from build123d import *

# Parameters (mm, degrees)
F1_DEPTH = 26
F2_R     = 3
F3_DEPTH = 25
F4_R     = 3
F5_DEPTH = 25
F6_R     = 4
F7_R     = 0.5


with BuildPart() as f1:
    # F0 (on Front) → F1 (new body)
    with BuildSketch(Plane.XZ):
        Polygon((0, 0), (0, 33.5), (-6.5, 33.5), (-6.5, -6.5), (19.5, -6.5), (19.5, 0), align=None)
    extrude(amount=-F1_DEPTH)

    # F2 (on Right) → F3 (cut)
    with BuildSketch(Plane.YZ):
        with Locations((13, 23.5)):
            Circle(F2_R)
    extrude(amount=-F3_DEPTH, mode=Mode.SUBTRACT)

    # F4 (on Top) → F5 (cut)
    with BuildSketch(Plane.XY):
        with Locations((6.5, 13)):
            Circle(F4_R)
    extrude(amount=-F5_DEPTH, mode=Mode.SUBTRACT)

    # F6
    f6_edges = [f1.edges().sort_by_distance(p)[0] for p in [
        (-6.5, 13, 33.5),
        (19.5, 13, 0),
    ]]
    fillet(f6_edges, radius=F6_R)

    # F7
    f7_edges = [f1.edges().sort_by_distance(p)[0] for p in [
        (-6.5, 0, 11.5),
        (-6.5, 26, 11.5),
        (7.75, 26, 0),
        (0, 26, 16.75),
        (0, 0, 16.75),
        (7.75, 0, 0),
    ]]
    fillet(f7_edges, radius=F7_R)


solid = f1.part
Work out the finished part from the listing and answer in its coordinate system (mm). A direction names the side the tool comes from. Round coordinates to 2 decimals unless told otherwise and drop trailing zeros. Loops run counter-clockwise (first coordinate to the right, second up) from the corner with the lowest first, then second, coordinate; pieces in that order, holes last. Notation, with made-up numbers: (-3.75, 80.5) - (29.25, 80.5) arc R33 cw to (29.25, 117.5) - close; hole circle Ø10 at (61, 4.25). An arc over 180 degrees is marked (long way). One line per item, written item: value.
Q1. Find section B-B on x = 6.5. Give the vertices of the cut face in (y, z), and give its area (3 significant figures).
Check values:
outline: (0, -6.5) - (10, -6.5) - (10, 0) - (0.5, 0) arc R0.5 ccw to (0, -0.5) - close; (16, -6.5) - (26, -6.5) - (26, -0.5) arc R0.5 ccw to (25.5, 0) - (16, 0) - close
area: 130 mm2
Q2. Straight lines are drawn through the part: probe 1 along Z at (x, y) = (-2.25, 13); probe 2 along Y at (x, z) = (6.5, -2.25); probe 3 along Z at (x, y) = (7, 22). For each, find the intervals that lie inside material, in ascending order.
Check values:
probe 1: -6.5 to 20.5, 26.5 to 33.5
probe 2: 0 to 10, 16 to 26
probe 3: -6.5 to 0
Q3. Find section C-C on z = 23.5. Give the vertices of the cut face in (x, y), and give its area (3 significant figures).
Check values:
outline: (-6.5, 0.5) arc R0.5 ccw to (-6, 0) - (-0.5, 0) arc R0.5 ccw to (0, 0.5) - (0, 10) - (-6.5, 10) - close; (-6.5, 16) - (0, 16) - (0, 25.5) arc R0.5 ccw to (-0.5, 26) - (-6, 26) arc R0.5 ccw to (-6.5, 25.5) - close
area: 130 mm2
Q4. Find section A-A on y = 13. Give the vertices of the cut face in (x, z), and give its area (3 significant figures).
Check values:
outline: (-6.5, -6.5) - (3.5, -6.5) - (3.5, 0) - (0, 0) - (0, 20.5) - (-6.5, 20.5) - close; (-6.5, 26.5) - (0, 26.5) - (0, 33.5) - (-2.5, 33.5) arc R4 ccw to (-6.5, 29.5) - close; (9.5, -6.5) - (19.5, -6.5) - (19.5, -4) arc R4 ccw to (15.5, 0) - (9.5, 0) - close
area: 302 mm2
Q5. For faces 4 (the flat face through (10, 13, 0)), 5 (the cylindrical face through (-5.297, 13.175, 32.359)), determine the directions among +Z, -Z, +X, -X, +Y, -Y from which every point of the face is accessible in a straight line to the end or side of a thin tool.
Check values:
face 4: +Z, +X, +Y, -Y
face 5: +Z, -X, +Y, -Y
Q6. Find section D-D on x = -1.75. Give the vertices of the cut face in (y, z), and give its area (3 significant figures).
Check values:
outline: (0, -6.5) - (26, -6.5) - (26, 33) arc R0.5 ccw to (25.5, 33.5) - (0.5, 33.5) arc R0.5 ccw to (0, 33) - close; hole circle Ø6 at (13, 23.5)
area: 1,010 mm2
Q7. Each of these flat-tipped pins is pushed along its axis until it touches: pin 1 Ø8 at (x, y) = (7, 11) entering from +Z; pin 2 Ø3 at (y, z) = (3.5, 20.5) entering from +X; pin 3 Ø6 at (x, z) = (0, 1.5) entering from +Y. Where does it stop, or does it pass through?
Check values:
pin 1: z = 0
pin 2: x = 0
pin 3: y = 26
Q8. The mould has two halves that part along Y. Classify faces 1 (the cylindrical face through (9.27, 11.85, -3.2)), 2 (the flat face through (-1, 26, 6)), 3 (the flat face through (3, 13, -6.5)): +Y half, -Y half, draft (parallel to the pull), parting line (faces both ways), or undercut.
Check values:
face 1: undercut
face 2: +Y half
face 3: draft
